Check sheet for the modelled part. Datum: model origin and axes. Units: mm. Give positions to 0.01 mm unless a question says otherwise; leave off trailing zeros. Order: outer loops, then holes, each group sorted by start corner. A loop starts at its lowest first (then second) coordinate and runs counter-clockwise, first axis right, second up.
```python
from build123d import *

# Parameters (mm, degrees)
BOSS_EXTRUDE1_DEPTH = 29.464
SKETCH2_R           = 3
CUT_EXTRUDE1_DEPTH  = 254


with BuildPart() as part:
    # Sketch1 → Boss-Extrude1 (new body)
    with BuildSketch(Plane(origin=(0, 0, 0), x_dir=(1, 0, 0), z_dir=(0, 1, 0))):
        with BuildLine():
            ThreePointArc((1.117349967, -6.351558659), (2.390405172, -4.153620888), (4.93040272, -4.15715015))
            Line((4.93040272, -4.15715015), (6.059286136, -2.208125873))
            ThreePointArc((6.059286136, -2.208125873), (4.792343793, -0.00665884), (6.065398997, 2.191278931))
            Line((6.065398997, 2.191278931), (4.941936169, 4.143432786))
            ThreePointArc((4.941936169, 4.143432786), (2.401938621, 4.146962048), (1.134996277, 6.348429081))
            Line((1.134996277, 6.348429081), (-1.117349967, 6.351558659))
            ThreePointArc((-1.117349967, 6.351558659), (-2.390405172, 4.153620888), (-4.93040272, 4.15715015))
            Line((-4.93040272, 4.15715015), (-6.059286136, 2.208125873))
            ThreePointArc((-6.059286136, 2.208125873), (-5.13175503, 1.27865958), (-4.792341341, 0.010188102))
            ThreePointArc((-4.792341341, 0.010188102), (-5.133519662, -1.261339807), (-6.065398997, -2.191278931))
            Line((-6.065398997, -2.191278931), (-4.941936169, -4.143432786))
            ThreePointArc((-4.941936169, -4.143432786), (-2.403465916, -4.14607814), (-1.134993825, -6.344899819))
            ThreePointArc((-1.134993825, -6.344899819), (-1.134994438, -6.346664451), (-1.134996277, -6.348429081))
            Line((-1.134996277, -6.348429081), (1.117349967, -6.351558659))
        make_face()
    extrude(amount=BOSS_EXTRUDE1_DEPTH)

    # Sketch2 → Cut-Extrude1 (cut)
    with BuildSketch(Plane(origin=(0, 29.464, 0), x_dir=(1, 0, 0), z_dir=(0, 1, 0))):
        Circle(SKETCH2_R)
    extrude(amount=-CUT_EXTRUDE1_DEPTH, mode=Mode.SUBTRACT)


solid = part.part
```
(1) Release check for a two-part mould opening along X. For faces 1 (the face through (-2.436, 14.526, 4.128)), 2 (the face through (-3, 15, 0)), 3 (the face through (-3, 0, -2)), 4 (the face through (-5.487, 14.526, -3.196)) record: released by +X, released by -X, zero draft, split by the parting line, or undercut.
Response values:
face 1: undercut
face 2: undercut
face 3: zero draft
face 4: released by -X
(2) Material ranges on L1, parallel to X at y = 8, z = 0; L2, parallel to Z at x = 0, y = 17.5; L3, parallel to Z at x = 3.5, y = 14.25, recorded low to high.
Response values:
L1: x = -4.79 to -3, 3 to 4.79
L2: z = -6.35 to -3, 3 to 6.35
L3: z = -3.81 to 3.82
(3) Cross-section at A-A on x = 0. Enter the section's corners in (y, z).
Response values:
outline: (0, -6.35) - (29.46, -6.35) - (29.46, -3) - (0, -3) - close; (0, 3) - (29.46, 3) - (29.46, 6.35) - (0, 6.35) - close
(4) Cross-section at D-D on x = 3.5. Enter the section's corners in (y, z), then the cut area to 3 significant figures.
Response values:
outline: (0, -3.81) - (29.46, -3.81) - (29.46, 3.82) - (0, 3.82) - close
area: 225 mm2
(5) Gauge pin test, flat ends, axial feed: pin 1 Ø3 at (x, y) = (4, 10.5) entering from -Z; pin 2 Ø2 at (y, z) = (25, 2) entering from -X; pin 3 Ø2 at (y, z) = (24, -0.5) entering from -X. Record the tip position at first contact, or that the pin passes through.
Response values:
pin 1: stops at z = -4.14
pin 2: stops at x = -6.07
pin 3: stops at x = -5.28
(6) Cross-section at C-C on z = -1. Enter the section's corners in (x, y), then the cut area to 3 significant figures.
Response values:
outline: (-4.99, 0) - (-2.83, 0) - (-2.83, 29.46) - (-4.99, 29.46) - close; (2.83, 0) - (5, 0) - (5, 29.46) - (2.83, 29.46) - close
area: 128 mm2
